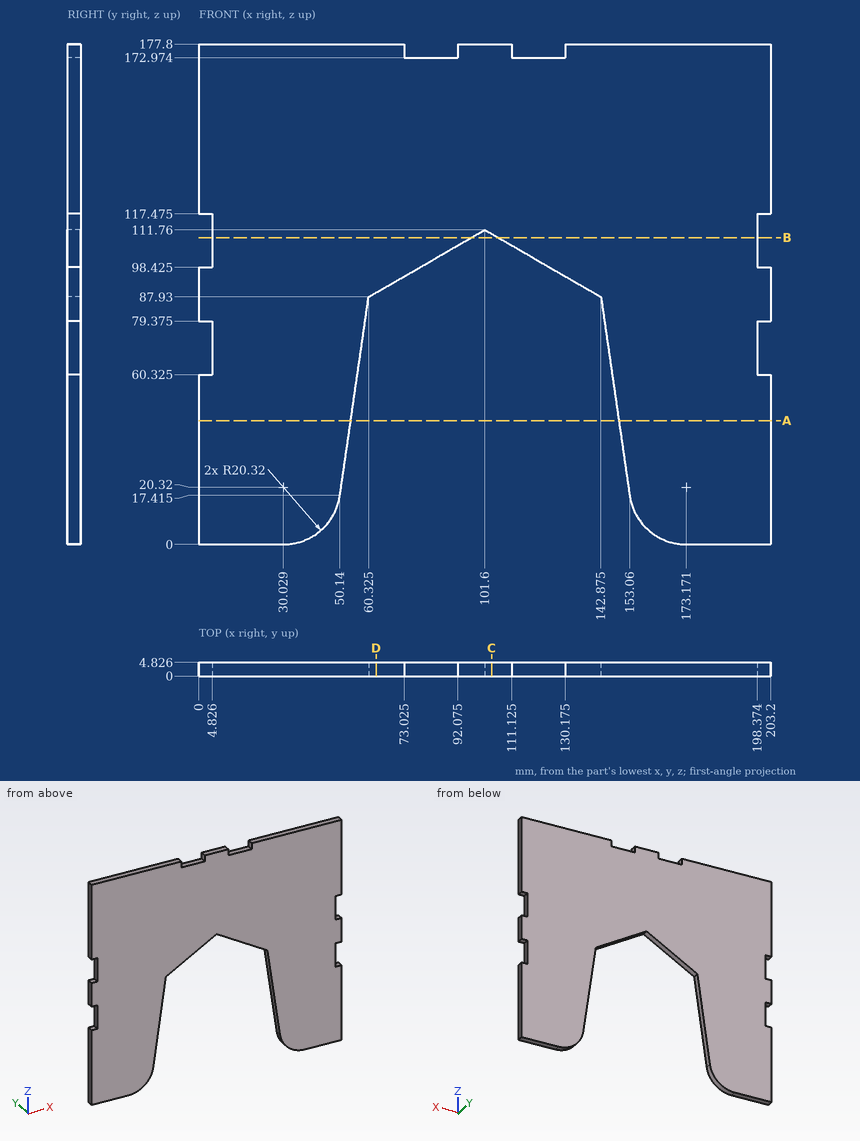
Print and shaded views of the part. All mm, measured from the part's lowest x, y and z. Give positions to 0.01 mm unless a question says otherwise; leave off trailing zeros. Write each loop counter-clockwise with the first axis right and the second up, starting at its lowest first coordinate (ties: lowest second). Pieces come first, ordered by that corner, then holes. Notation, with made-up numbers: (-11, 18.5) -> (4, 18.5) arc R21 ccw to (4, 56.5) -> close; hole circle Ø7 at (75.5, 15.5). An arc over 180 degrees is marked (long way). Use CSV: the item, a comma, the result in double quotes. Start each with the question number.
1) Cut at A-A on z = 44. List the corners of the cut face in (x, y).
2) Cut at C-C on x = 104. List the corners of the cut face in (y, z) (1 decimal).
3) Cut at D-D on x = 63. List the corners of the cut face in (y, z), plus the area to 3 significant figures.
4) Pin check, flat tips, straight feed: P1, Ø2.5, axis at x = 117.5, y = 3, coming from the +Z side; P2, Ø1, axis at x = 76.5, y = 3.5, coming from the -Z side; P3, Ø1.4, axis at y = 2, z = 104.5, coming from the -X side. Stop position of each tip, or through.
5) Drill centre lines: L1, parallel to X at y = 2.25, z = 13 (1 decimal); L2, parallel to X at y = 4.5, z = 98 (1 decimal); L3, parallel to Z at x = 139, y = 1.45. Where is each one in solid material? Low to high.
6) Cut at B-B on z = 109. List the corners of the cut face in (x, y).
Final values:
1,outline,"(0, 0) -> (53.98, 0) -> (53.98, 4.83) -> (0, 4.83) -> close; (149.22, 0) -> (203.2, 0) -> (203.2, 4.83) -> (149.22, 4.83) -> close"
2,outline,"(0, 110.4) -> (4.8, 110.4) -> (4.8, 177.8) -> (0, 177.8) -> close"
3,outline,"(0, 89.47) -> (4.83, 89.47) -> (4.83, 177.8) -> (0, 177.8) -> close"
3,area,"426 mm2"
4,P1,"stops at z = 172.97"
4,P2,"stops at z = 96.98"
4,P3,"stops at x = 4.83"
5,L1,"x = 0 to 49, 154.2 to 203.2"
5,L2,"x = 0 to 77.8, 125.4 to 203.2"
5,L3,"z = 90.17 to 177.8"
6,outline,"(4.83, 0) -> (96.82, 0) -> (96.82, 4.83) -> (4.83, 4.83) -> close; (106.38, 0) -> (198.37, 0) -> (198.37, 4.83) -> (106.38, 4.83) -> close"
